Drawing for the job (mm, zero at the part's lowest x, y, z). A direction names the side the tool comes from. Give positions to 0.01 mm unless a question says otherwise; leave off trailing zeros. Loops run counter-clockwise (first coordinate to the right, second up) from the corner with the lowest first, then second, coordinate; pieces in that order, holes last. Notation, with made-up numbers: (19, 66) - (78, 66) arc R10 cw to (78, 70) - close; hole circle Ø8 at (-17, 4.5). An arc over 180 degrees is marked (long way). Return JSON: item names as keys, results as strings. Group by question number.
1) Slice it at C-C (z = 2.25). List the corners of the cut face in (x, y) (3 decimals).
2) Slice it at D-D (z = 12.5). List the corners of the cut face in (x, y).
3) Slice it at A-A (y = 4). List the corners of the cut face in (x, z) (3 decimals).
4) Drop flat-ended pins along their axis: pin 1 (2 mm diameter, centred on y = 6.5, z = 17, fed in from +X); pin 2 (1.8 mm diameter, centred on x = 3.5, y = 4, fed in from +Z); pin 3 (1.5 mm diameter, centred on x = 6.5, z = 13, fed in from +Y). Give the stop position or say it passes through.
5) Mould opens along X. For the marked faces 1, 2 and 3 say: released by +X, released by -X, zero draft, split by the parting line, or undercut.
6) 3-axis set-ups, long thin cutter, end or side, ignore diameter. For the marked faces 4 and 5: which of +Z, -Z, +X, -X, +Y, -Y reach the whole face in a straight line?
7) Drill centre lines: probe 1 along Y at (x, z) = (4, 15.5); probe 2 along Z at (x, y) = (5, 4.75); probe 3 along Y at (x, z) = (4, 3.5) (3 decimals). Where is each one in solid material? Low to high. Write a range as from..to.
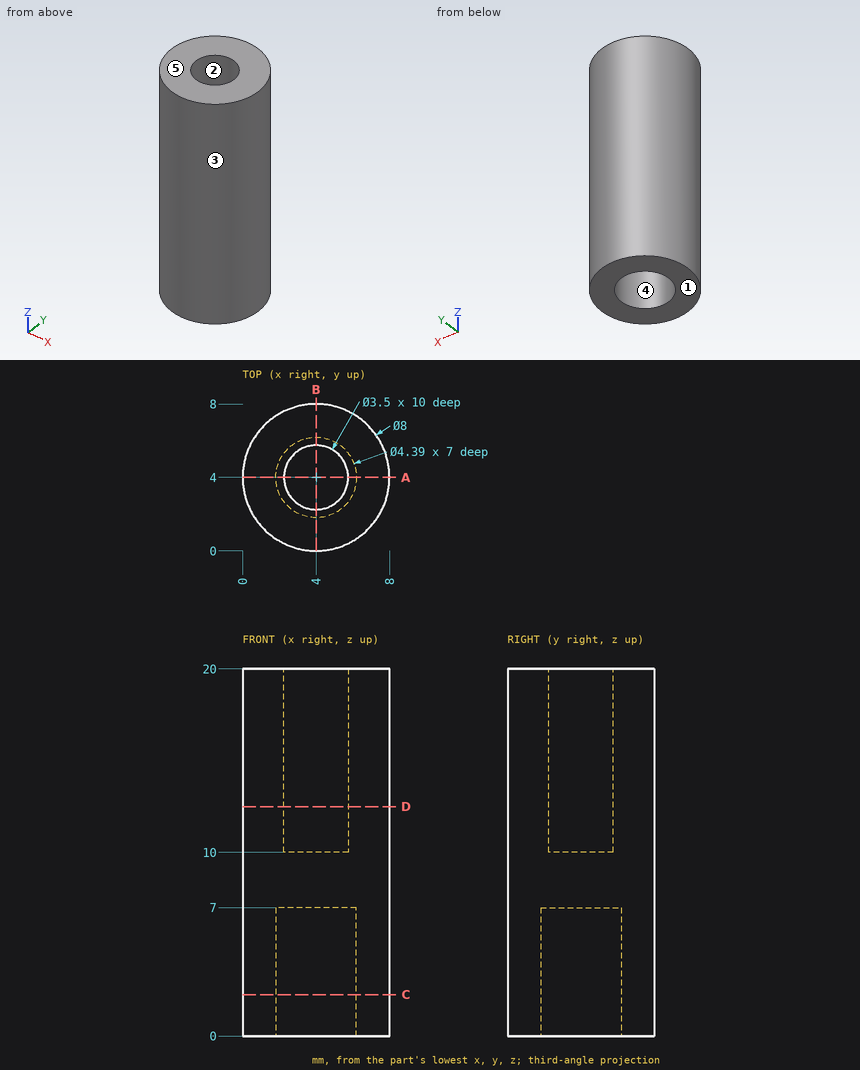
Results:
{
 "1": {"outline": "circle Ø8 at (4, 4); hole circle Ø4.39 at (4, 4)"},
 "2": {"outline": "circle Ø8 at (4, 4); hole circle Ø3.5 at (4, 4)"},
 "3": {"outline": "(0, 0) - (1.805, 0) - (1.805, 7) - (6.195, 7) - (6.195, 0) - (8, 0) - (8, 20) - (5.75, 20) - (5.75, 10) - (2.25, 10) - (2.25, 20) - (0, 20) - close"},
 "4": {"pin 1": "x = 7.71", "pin 2": "z = 10", "pin 3": "y = 7.6"},
 "5": {"face 1": "zero draft", "face 2": "undercut", "face 3": "split by the parting line"},
 "6": {"face 4": "-Z", "face 5": "+Z, +X, -X, +Y, -Y"},
 "7": {"probe 1": "0..2.25, 5.75..8", "probe 2": "7..10", "probe 3": "0..1.805, 6.195..8"}
}
